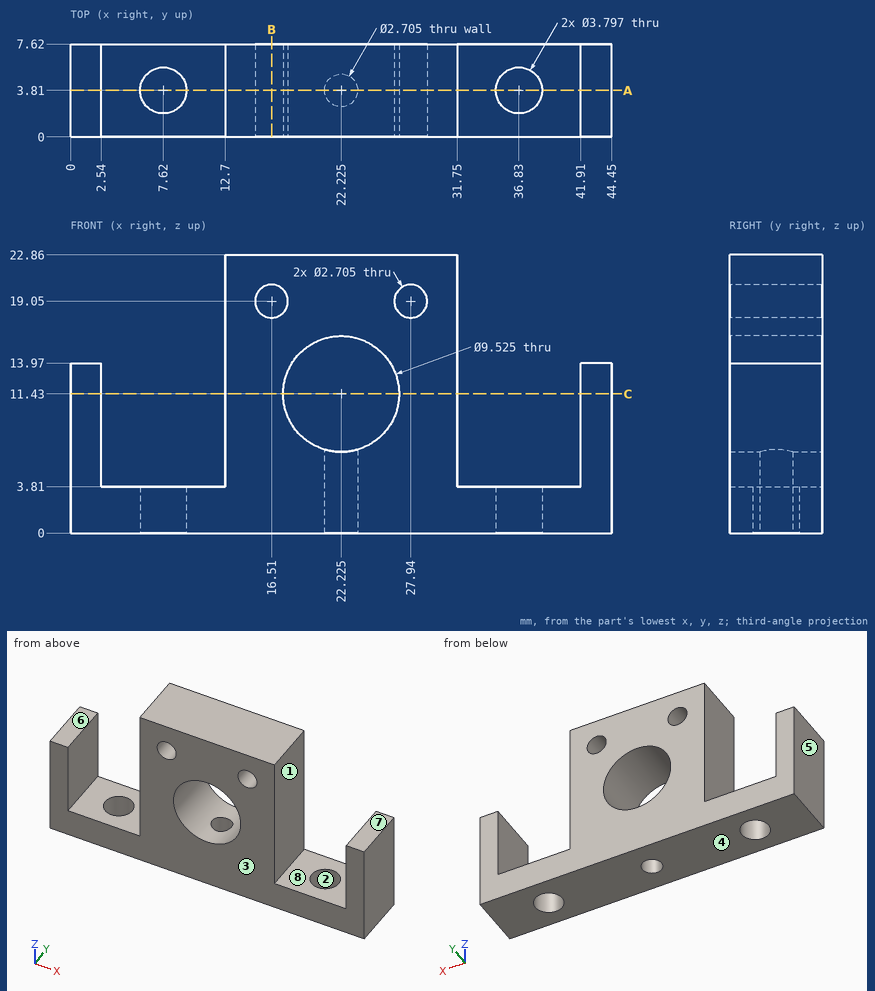
Geometry check sheet. Reference: drawing and pictorial views, mm from the part's lowest x, y, z. A direction names the side the tool comes from. Coordinates: 2 decimals unless noted, no trailing zeros. Loops run counter-clockwise (first coordinate to the right, second up) from the corner with the lowest first, then second, coordinate; pieces in that order, holes last.
1) Material ranges on probe 1 along X at (y, z) = (1.5, 11.43); probe 2 along X at (y, z) = (0.75, 5); probe 3 along X at (y, z) = (1, 19), recorded low to high.
2) Access from +Z, -Z, +X, -X, +Y, -Y to the whole of each face (thin tool, end or side, straight path). Record for the marked faces 4, 5, 6, 7 and 8.
3) Release check for a two-part mould opening along Y. For the marked faces 1, 2 and 3 record: released by +Y, released by -Y, zero draft, split by the parting line, or undercut.
4) Sectioned sample at B-B (x = 16.51). Record the boundary of the cut face in (y, z).
5) Gauge pin test, flat ends, axial feed: pin 1 (4.5 mm diameter, centred on x = 7.62, y = 3.81, fed in from +Z); pin 2 (1.3 mm diameter, centred on x = 43.5, y = 2.5, fed in from +Z); pin 3 (1.5 mm diameter, centred on y = 3, z = 19, fed in from -X). Record the tip position at first contact, or that the pin passes through.
6) Sectioned sample at C-C (z = 11.43). Record the boundary of the cut face in (x, y), and give its area (3 significant figures).
7) Sectioned sample at A-A (y = 3.81). Count the separate pieces of the cut face and the enclosed holes in it, and give its area (3 significant figures).
Check sheet entries:
1. probe 1: x = 0 to 2.54, 12.7 to 17.46, 26.99 to 31.75, 41.91 to 44.45
1. probe 2: x = 0 to 2.54, 12.7 to 31.75, 41.91 to 44.45
1. probe 3: x = 12.7 to 15.16, 17.86 to 26.59, 29.29 to 31.75
2. face 4: -Z, +X, -X, +Y, -Y
2. face 5: +Z, -Z, -X, +Y, -Y
2. face 6: +Z, -X, +Y, -Y
2. face 7: +Z, +X, +Y, -Y
2. face 8: +Z, +Y, -Y
3. face 1: zero draft
3. face 2: undercut
3. face 3: released by -Y
4. outline: (0, 0) - (7.62, 0) - (7.62, 17.7) - (0, 17.7) - close; (0, 20.4) - (7.62, 20.4) - (7.62, 22.86) - (0, 22.86) - close
5. pin 1: stops at z = 3.81
5. pin 2: stops at z = 13.97
5. pin 3: stops at x = 12.7
6. outline: (0, 0) - (2.54, 0) - (2.54, 7.62) - (0, 7.62) - close; (12.7, 0) - (17.46, 0) - (17.46, 7.62) - (12.7, 7.62) - close; (26.99, 0) - (31.75, 0) - (31.75, 7.62) - (26.99, 7.62) - close; (41.91, 0) - (44.45, 0) - (44.45, 7.62) - (41.91, 7.62) - close
6. area: 111 mm2
7. separate pieces: 3
7. enclosed holes: 2
7. area: 454 mm2
